Build history of the part. All positions in model axes, mm. A direction names the side the tool comes from. Round coordinates to 2 decimals unless told otherwise and drop trailing zeros. Loops run counter-clockwise (first coordinate to the right, second up) from the corner with the lowest first, then second, coordinate; pieces in that order, holes last. Notation, with made-up numbers: (29.25, 9.5) -> (87.25, 9.5) arc R13 ccw to (87.25, 20.5) -> close; hole circle Ø5 at (-34, 42.5). An arc over 180 degrees is marked (long way). Put each result on its own line as item: value. Start each with the question number.
Item 1: Cut at B-B, the plane x = -71. List the corners of the cut face in (y, z).
Item 2: Pull direction Z, two halves, no side cores. Call faces 6 (the flat face through (4, -11, 25.4)), 7 (the cylindrical face through (-30.299, -82.165, 0.371)), 8 (the flat face through (20.246, -69, 1)): +Z half, -Z half, draft (parallel to the pull), parting line (faces both ways), or undercut.
Item 3: Drill centre lines: probe 1 along X at (y, z) = (-13, 10); probe 2 along X at (y, z) = (-73.5, 6.5); probe 3 along Y at (x, z) = (-43.5, -11.5). Where is each one in solid material? Low to high. Write a range as [from, to].
Item 4: Cut at C-C, the plane z = 15.5. List the corners of the cut face in (x, y).
Item 5: Cut at A-A, the plane y = -14. List the corners of the cut face in (x, z), plus the area to 3 significant figures.
Item 6: Tool access for faces 1 (the flat face through (-23.113, -70, 1)), 2 (the flat face through (-37.286, -64, 1)), 3 (the flat face through (24, -55, 20.064)), 4 (the flat face through (37.286, -64, 2)), 5 (the cylindrical face through (28.885, -98.275, 0.49)): list every direction of +Z, -Z, +X, -X, +Y, -Y with a clear straight run to the whole face (end or side of a thin tool).
Item 7: Flat gauge pins, fed straight in: pin 1 Ø8 at (y, z) = (-54.5, 10) entering from +X; pin 2 Ø20 at (y, z) = (-87.13, 0) entering from +X; pin 3 Ø8 at (x, z) = (23.5, 12.5) entering from -Y. Where does each tip first touch, or does it go through?
Item 8: Cut at D-D, the plane y = -37.5. List the corners of the cut face in (x, z).
```python
from build123d import *

# Parameters (mm, degrees)
F0_R      = 12.7
F1_DEPTH  = 22.606
F2_W      = 74.5722576976
F2_H      = 22.3488807678
F3_DEPTH  = 83.312
F4_DEPTH  = 5.588
F5_DEPTH  = 8.89
F7_DEPTH  = 127.254
F8_R      = 8.4373748016
F9_DEPTH  = 25.4
F10_R     = 11.1555732281
F11_DEPTH = 25.4
F12_R     = 17.78
F13_R     = 17.78


with BuildPart() as f1:
    # F0 (on Front) → F1 (new body)
    with BuildSketch(Plane.XZ):
        with BuildLine():
            Line((82.5530235944, 25.4), (-77.1982306158, 25.4))
            ThreePointArc((-77.1982306158, 25.4), (-102.5982306158, 0), (-77.1982306158, -25.4))
            Line((-77.1982306158, -25.4), (82.5530235944, -25.4))
            ThreePointArc((82.5530235944, -25.4), (107.9530235944, 0), (82.5530235944, 25.4))
        make_face()
        with Locations((-77.1982306158, 0)):
            Circle(F0_R, mode=Mode.SUBTRACT)
        with Locations((82.5530235944, 0)):
            Circle(F0_R, mode=Mode.SUBTRACT)
    extrude(amount=F1_DEPTH)

    # F2 (on face) → F3 (join)
    with BuildSketch(Plane.XZ.offset(22.606)):
        Rectangle(F2_W, F2_H)
    extrude(amount=F3_DEPTH)

    # F4 (add): a face of the model
    f4_faces = [f1.faces().sort_by_distance(p)[0] for p in [
        (0, -64.262, -11.1744403839),
    ]]
    extrude(f4_faces, amount=F4_DEPTH)

    # F5 (add): a face of the model
    f5_faces = [f1.faces().sort_by_distance(p)[0] for p in [
        (0, -64.262, 11.1744403839),
    ]]
    extrude(f5_faces, amount=F5_DEPTH)

    # F6 (on face) → F7 (cut)
    with BuildSketch(Plane(origin=(0, 0, -16.7624403839), x_dir=(1, 0, 0), z_dir=(0, 0, -1))):
        with BuildLine():
            Line((20.2462481307, 105.918), (-23.1126956642, 105.918))
            Line((-23.1126956642, 105.918), (-23.1126956642, 46.0643023252))
            ThreePointArc((-23.1126956642, 46.0643023252), (-1.4332237667, 24.3848304278), (20.2462481307, 46.0643023252))
            Line((20.2462481307, 46.0643023252), (20.2462481307, 105.918))
        make_face()
    extrude(amount=-F7_DEPTH, mode=Mode.SUBTRACT)

    # F8 (on face) → F9 (cut)
    with BuildSketch(Plane(origin=(-37.2861288488, 0, 0), x_dir=(0, -1, 0), z_dir=(-1, 0, 0))):
        with Locations((90.5945748091, 0)):
            Circle(F8_R)
    extrude(amount=-F9_DEPTH, mode=Mode.SUBTRACT)

    # F10 (on face) → F11 (cut)
    with BuildSketch(Plane.YZ.offset(37.2861288488)):
        with Locations((-87.1303528547, 0)):
            Circle(F10_R)
    extrude(amount=-F11_DEPTH, mode=Mode.SUBTRACT)

    # F12
    f12_edges = [f1.edges().sort_by_distance(p)[0] for p in [
        (-30.199412, -105.918, -16.76244),
        (-30.199412, -105.918, 20.06444),
    ]]
    fillet(f12_edges, radius=F12_R)

    # F13
    f13_edges = [f1.edges().sort_by_distance(p)[0] for p in [
        (28.766188, -105.918, 20.06444),
        (28.766188, -105.918, -16.76244),
    ]]
    fillet(f13_edges, radius=F13_R)


solid = f1.part
```
Reply:
1. outline: (-22.61, -25.4) -> (0, -25.4) -> (0, -11.08) -> (-22.61, -11.08) -> close; (-22.61, 11.08) -> (0, 11.08) -> (0, 25.4) -> (-22.61, 25.4) -> close
2. face 6: +Z half
2. face 7: undercut
2. face 8: draft
3. probe 1: x = [-100.55, -85.03], [-69.37, 74.72], [90.38, 105.9]
3. probe 2: x = [-37.29, -23.11], [20.25, 37.29]
3. probe 3: y = [-22.61, 0]
4. outline: (-97.32, -22.61) -> (-37.29, -22.61) -> (-37.29, -100.03) -> (-23.11, -100.03) -> (-23.11, -46.06) arc R21.68 cw to (20.25, -46.06) -> (20.25, -100.03) -> (37.29, -100.03) -> (37.29, -22.61) -> (102.68, -22.61) -> (102.68, 0) -> (-97.32, 0) -> close
5. outline: (-77.2, -25.4) -> (82.55, -25.4) arc R25.4 ccw to (82.55, 25.4) -> (-77.2, 25.4) arc R25.4 ccw to start; hole circle Ø25.4 at (-77.2, 0); hole circle Ø25.4 at (82.55, 0)
5. area: 9,130 mm^2
6. face 1: +Z, -Z, -Y
6. face 2: +Z, -Z, -X, -Y
6. face 3: +Z, +X, -X, -Y
6. face 4: +Z, -Z, +X, -Y
6. face 5: +X
7. pin 1: stops at x = 37.29
7. pin 2: stops at x = -23.11
7. pin 3: stops at y = -104.8
8. outline: (-37.29, -16.76) -> (-21.35, -16.76) -> (-21.35, 20.06) -> (-37.29, 20.06) -> close; (18.48, -16.76) -> (37.29, -16.76) -> (37.29, 20.06) -> (18.48, 20.06) -> close
